Can you work these out from the drawing? Everything is in mm from the part's minimum corner. Coordinates: 2 decimals unless noted, no trailing zeros. Loops run counter-clockwise (first coordinate to the right, second up) from the corner with the lowest first, then second, coordinate; pieces in that order, holes last.
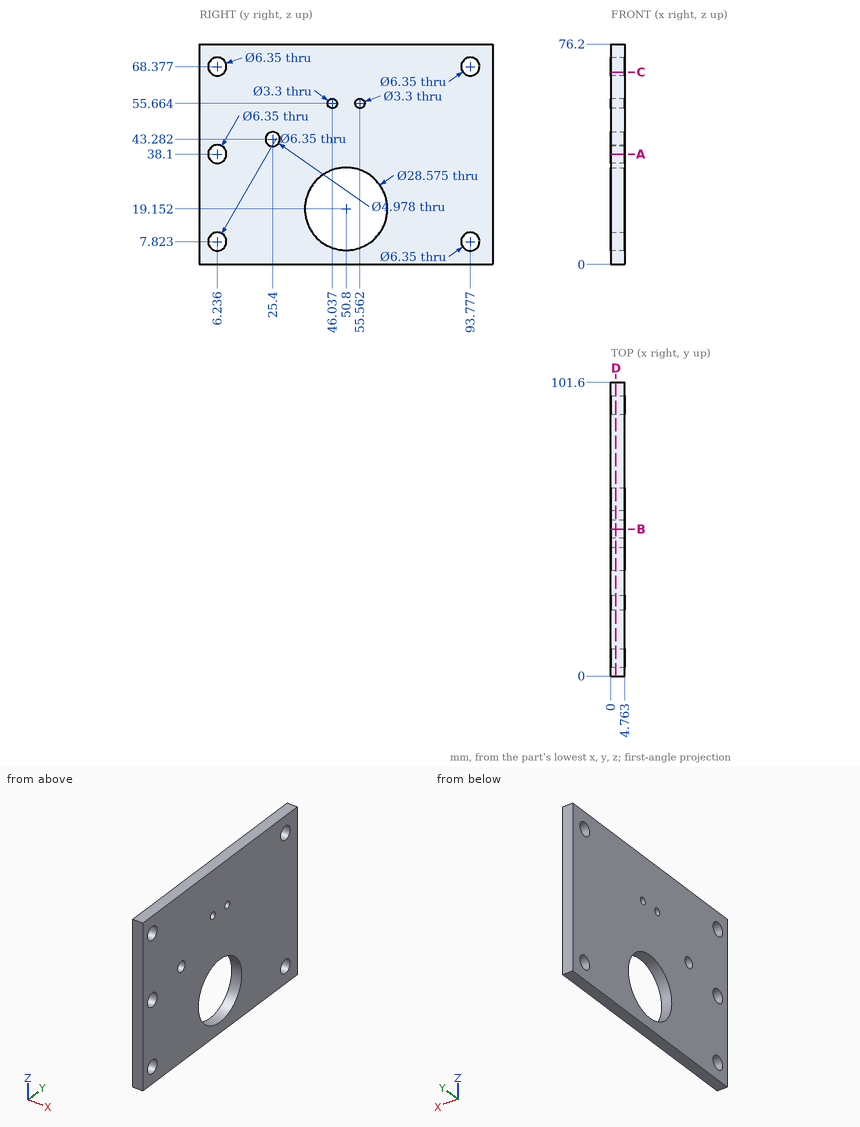
1. For pin 1 (4 mm diameter, centred on y = 25.4, z = 43.28, fed in from -X), with a flat end and sliding along its axis, tell me the tip position at first contact or that it passes through.
2. I want a section at D-D (x = 1.7). Give the number of separate pieces and of enclosed holes in the cut face, then the cut area to 3 significant figures.
3. I want a section at B-B (y = 50.8). Please give me the cut outline in (x, z) (1 decimal).
4. I need wall thicknesses on line 1 along Y through (x, z) = (3.25, 55.5) (1 decimal); line 2 along Z through (x, y) = (2.2, 45.5) (1 decimal); line 3 along Y through (x, z) = (2.8, 6) (1 decimal). Which ranges of each line are inside material? Lowest first, please.
5. I want a section at C-C (z = 66.5). Please give me the cut outline in (x, y) (1 decimal), then the cut area to 3 significant figures.
6. I want a section at A-A (z = 38.1). Please give me the cut outline in (x, y).
Response values:
1. pin 1: passes through
2. separate pieces: 1
2. enclosed holes: 9
2. area: 6,910 mm2
3. outline: (0, 0) - (4.8, 0) - (4.8, 4.9) - (0, 4.9) - close; (0, 33.4) - (4.8, 33.4) - (4.8, 76.2) - (0, 76.2) - close
4. line 1: y = 0 to 44.4, 47.7 to 53.9, 57.2 to 101.6
4. line 2: z = 0 to 5.9, 32.4 to 54.1, 57.2 to 76.2
4. line 3: y = 0 to 3.6, 8.8 to 45.2, 56.4 to 91.2, 96.4 to 101.6
5. outline: (0, 0) - (4.8, 0) - (4.8, 3.7) - (0, 3.7) - close; (0, 8.8) - (4.8, 8.8) - (4.8, 91.2) - (0, 91.2) - close; (0, 96.3) - (4.8, 96.3) - (4.8, 101.6) - (0, 101.6) - close
5. area: 435 mm2
6. outline: (0, 0) - (4.76, 0) - (4.76, 3.06) - (0, 3.06) - close; (0, 9.41) - (4.76, 9.41) - (4.76, 101.6) - (0, 101.6) - close
